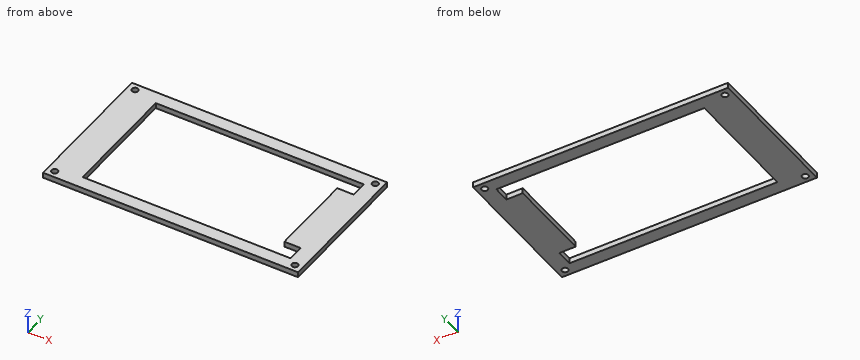
```python
from build123d import *

# Parameters (mm, degrees)
SKETCH_1_W          = 140.7
SKETCH_1_H          = 78.95
SKETCH_1_R          = 1.7
EXTRUDE_1_DEPTH     = 3
SKETCH_2_W          = 105.7
SKETCH_2_H          = 64.95
CUT_EXTRUDE_1_DEPTH = 81.724210278
SKETCH_3_W          = 9
SKETCH_3_H          = 9
CUT_EXTRUDE_2_DEPTH = 81.724210278


with BuildPart() as part:
    # 草图1 → 凸台-拉伸1 (new body)
    with BuildSketch(Plane.XY):
        Rectangle(SKETCH_1_W, SKETCH_1_H)
        with Locations((-66.25272379, 35.66826865)):
            Circle(SKETCH_1_R, mode=Mode.SUBTRACT)
        with Locations(Location((66.25272379, 35.66826865, 0), (0, 0, 180))):
            Circle(SKETCH_1_R, mode=Mode.SUBTRACT)
        with Locations((66.25272379, -35.66826865)):
            Circle(SKETCH_1_R, mode=Mode.SUBTRACT)
        with Locations(Location((-66.25272379, -35.66826865, 0), (0, 0, 180))):
            Circle(SKETCH_1_R, mode=Mode.SUBTRACT)
    extrude(amount=EXTRUDE_1_DEPTH)

    # 草图2 → 切除-拉伸1 (cut, through all)
    with BuildSketch(Plane.XY.offset(3)):
        Rectangle(SKETCH_2_W, SKETCH_2_H)
    extrude(amount=-CUT_EXTRUDE_1_DEPTH, mode=Mode.SUBTRACT)

    # 草图3 → 切除-拉伸2 (cut, through all)
    with BuildSketch(Plane.XY.offset(3)):
        with Locations((57.35, 27.975)):
            Rectangle(SKETCH_3_W, SKETCH_3_H)
        with Locations((57.35, -27.975)):
            Rectangle(SKETCH_3_W, SKETCH_3_H)
    extrude(amount=-CUT_EXTRUDE_2_DEPTH, mode=Mode.SUBTRACT)


solid = part.part
```
Geometry check sheet. Reference: the model listing, model coordinates, mm. Give positions to 0.01 mm unless a question says otherwise; leave off trailing zeros. Order: outer loops, then holes, each group sorted by start corner. A loop starts at its lowest first (then second) coordinate and runs counter-clockwise, first axis right, second up.
1. Thickness scan on L1, parallel to Y at x = 61.5, z = 0.65 (3 decimals); L2, parallel to X at y = -11, z = 1.25; L3, parallel to X at y = -29.5, z = 1.7. Record the ranges inside material, lowest first.
2. Section check C-C, the plane z = 1.8. Enter the section's corners in (x, y) (3 decimals).
3. Section check A-A, the plane x = -9.5. Enter the section's corners in (y, z) (3 decimals), and give its area (3 significant figures).
4. Section check B-B, the plane y = 12. Enter the section's corners in (x, z), and give its area (3 significant figures).
Values follow:
1. L1: y = -39.475 to -32.475, -23.475 to 23.475, 32.475 to 39.475
1. L2: x = -70.35 to -52.85, 52.85 to 70.35
1. L3: x = -70.35 to -52.85, 61.85 to 70.35
2. outline: (-70.35, -39.475) - (70.35, -39.475) - (70.35, 39.475) - (-70.35, 39.475) - close; hole circle Ø3.4 at (-66.253, -35.668); hole circle Ø3.4 at (-66.253, 35.668); hole (-52.85, -32.475) - (61.85, -32.475) - (61.85, -23.475) - (52.85, -23.475) - (52.85, 23.475) - (61.85, 23.475) - (61.85, 32.475) - (-52.85, 32.475) - close; hole circle Ø3.4 at (66.253, -35.668); hole circle Ø3.4 at (66.253, 35.668)
3. outline: (-39.475, 0) - (-32.475, 0) - (-32.475, 3) - (-39.475, 3) - close; (32.475, 0) - (39.475, 0) - (39.475, 3) - (32.475, 3) - close
3. area: 42.0 mm2
4. outline: (-70.35, 0) - (-52.85, 0) - (-52.85, 3) - (-70.35, 3) - close; (52.85, 0) - (70.35, 0) - (70.35, 3) - (52.85, 3) - close
4. area: 105 mm2
